```python
from build123d import *

# Parameters (mm, degrees)
F1_DEPTH = 7.62
F2_R     = 6.9977
F3_DEPTH = 23.0124
F4_R     = 6.3373
F5_DEPTH = 14.5542
F6_SIZE  = 0.508


with BuildPart() as f1:
    # F0 (on Right) → F1 (new body)
    with BuildSketch(Plane.YZ):
        with BuildLine():
            ThreePointArc((0.488564857, 5.885255698), (4.3451208276, 3.9993568537), (5.9055, 0))
            Line((5.9055, 0), (35.9918, 0))
            ThreePointArc((35.9918, 0), (30.0525244802, 14.6370582333), (15.5932935183, 20.9970195081))
            ThreePointArc((15.5932935183, 20.9970195081), (15.6296763666, 20.4153544005), (15.6418109969, 19.8326788821))
            ThreePointArc((15.6418109969, 19.8326788821), (11.1244567157, 9.5352097506), (0.488564857, 5.885255698))
        make_face()
        with BuildLine():
            Line((35.9918, 0), (5.9055, 0))
            ThreePointArc((5.9055, 0), (4.3451208206, -3.9993568613), (0.4885648365, -5.8852556997))
            ThreePointArc((0.4885648365, -5.8852556997), (11.1244567081, -9.5352097437), (15.6418109969, -19.8326788821))
            ThreePointArc((15.6418109969, -19.8326788821), (15.6296763666, -20.4153544005), (15.5932935183, -20.9970195081))
            ThreePointArc((15.5932935183, -20.9970195081), (30.0525244802, -14.6370582333), (35.9918, 0))
        make_face()
        with BuildLine():
            Line((5.9055, 0), (2.54, 0))
            ThreePointArc((2.54, 0), (0, -2.54), (-2.54, 0))
            Line((-2.54, 0), (-5.9055, 0))
            ThreePointArc((-5.9055, 0), (-3.9993568613, -4.3451208206), (0.4885648365, -5.8852556997))
            ThreePointArc((0.4885648365, -5.8852556997), (4.3451208206, -3.9993568613), (5.9055, 0))
        make_face()
        with BuildLine():
            ThreePointArc((-2.54, 0), (0, 2.54), (2.54, 0))
            Line((2.54, 0), (5.9055, 0))
            ThreePointArc((5.9055, 0), (4.3451208276, 3.9993568537), (0.488564857, 5.885255698))
            ThreePointArc((0.488564857, 5.885255698), (-3.9993568537, 4.3451208276), (-5.9055, 0))
            Line((-5.9055, 0), (-2.54, 0))
        make_face()
    extrude(amount=F1_DEPTH)

    # F2 (on face) → F3 (join)
    with BuildSketch(Plane(origin=(0, 0, 0), x_dir=(0, -1, 0), z_dir=(-1, 0, 0))):
        with Locations((-11.0998, 0)):
            Circle(F2_R)
    extrude(amount=F3_DEPTH)

    # F4 (on face) → F5 (join)
    with BuildSketch(Plane(origin=(-23.0124, 0, 0), x_dir=(0, -1, 0), z_dir=(-1, 0, 0))):
        with Locations((-11.0998, 0)):
            Circle(F4_R)
    extrude(amount=F5_DEPTH)

    # F6
    f6_edges = [f1.edges().sort_by_distance(p)[0] for p in [
        (-37.5666, 17.4371, 0),
    ]]
    chamfer(f6_edges, length=F6_SIZE)


solid = f1.part
```
Source: CAD feature listing. Evaluate the final solid. Frame: model axes, mm. A direction names the side the tool comes from. Coordinates: 2 decimals unless noted, no trailing zeros. Loops run counter-clockwise (first coordinate to the right, second up) from the corner with the lowest first, then second, coordinate; pieces in that order, holes last. Notation, with made-up numbers: M 34.5,-7.5 L 71.5,-7.5 A27 ccw 71.5,19.5 Z; hole C 24,39 d5. An arc over 180 degrees is marked long. Put each result on its own line as item: value. Start each with the question number.
1) Pull-direction query (Y, two-part tool) for faces 1 (the face through (3.76, 0.33, 2.52)), 2 (the face through (0, 19, 0)), 3 (the face through (-29.94, 17.43, 0.28)); classes: pulls with the +Y half, pulls with the -Y half, needs draft (parallel to the pull), parting line crosses it, or undercut.
2) Cut plane D-D on y = 23.5. Return the cut outline in (x, z).
3) Cut plane B-B on x = -30.5. Return the cut outline in (y, z).
4) Reachability of faces 4 (the face through (-37.567, 11, 0)), 5 (the face through (-23.012, 17.4, 1.6)) from +Z, -Z, +X, -X, +Y, -Y: full face, straight path, thin tool, end or side. Return the list, or none.
5) Cut plane A-A on y = -1. Return the cut outline in (x, z).
6) Contact query for flat-ended pins moving along their axis: pin 1 Ø12 at (x, y) = (-26.5, 13.5) entering from -Z; pin 2 Ø12 at (x, z) = (-6.5, -5.5) entering from -Y; pin 3 Ø1 at (x, y) = (-8, 9) entering from -Z. Output: stop coordinate, or through.
7) Cut plane C-C on z = -11. Return the cut outline in (x, y).
8) Ray query, L1, parallel to Z at x = 3.25, y = 0; L2, parallel to X at y = 13, z = 11; L3, parallel to X at y = 8, z = 6. Return the intervals inside material, ascending. Write a range as from..to.
The answers:
1. face 1: undercut
1. face 2: needs draft
1. face 3: parting line crosses it
2. outline: M 0,-19.2 L 7.62,-19.2 L 7.62,19.2 L 0,19.2 Z
3. outline: C 11.1,0 d12.67
4. face 4: +Z, -Z, -X, +Y, -Y
4. face 5: -X
5. outline: M 0,-5.82 L 7.62,-5.82 L 7.62,-2.33 L 0,-2.33 Z; M 0,2.33 L 7.62,2.33 L 7.62,5.82 L 0,5.82 Z
6. pin 1: stops at z = -7
6. pin 2: stops at y = 4.1
6. pin 3: stops at z = -6.81
7. outline: M 0,12.5 L 7.62,12.5 L 7.62,32.88 L 0,32.88 Z
8. L1: z = -5.91..-2.54, 2.54..5.91
8. L2: x = 0..7.62
8. L3: x = -23.01..7.62
